from build123d import *

# Parameters (mm, degrees)
SKETCH5_W                = 5.15874
SKETCH5_H                = 60.071
SKETCH10_R               = 9.3345
BOSS_EXTRUDE1_DEPTH      = 31.75
CUT_EXTRUDE7_START       = 91.821
SKETCH8_R                = 12.7
CUT_EXTRUDE7_DEPTH       = 22.225
CUT_EXTRUDE9_DEPTH       = 93.765089454
CUT_EXTRUDE9_DEPTH_BACK  = 93.765089454
SKETCH11_W               = 2
SKETCH11_H               = 3
CUT_EXTRUDE10_DEPTH      = 93.765089454
CUT_EXTRUDE10_DEPTH_BACK = 93.765089454
SKETCH12_R               = 1.5875
CUT_EXTRUDE11_DEPTH      = 93.765089454
CUT_EXTRUDE11_DEPTH_BACK = 93.765089454
SKETCH13_R               = 1.5875


with BuildPart() as part:
    # Sketch5 → Revolve2 (revolve)
    with BuildSketch(Plane(origin=(0, 0, 0), x_dir=(1, 0, 0), z_dir=(0, 1, 0)), mode=Mode.PRIVATE) as revolve2_sk:
        with Locations((2.57937, -30.0355)):
            Rectangle(SKETCH5_W, SKETCH5_H)
    revolve(revolve2_sk.sketch.rotate(Axis((0, 0, 0), (0, 0, 1)), 180), axis=Axis((0, 0, 0), (0, 0, 1)))

    # Sketch10 → Boss-Extrude1 (add)
    with BuildSketch(Plane.XY.offset(60.071)):
        Circle(SKETCH10_R)
    extrude(amount=BOSS_EXTRUDE1_DEPTH)

    # Sketch8 → Cut-Extrude7 (cut)
    with BuildSketch(Plane.XY.offset(CUT_EXTRUDE7_START)):
        Circle(SKETCH8_R)
        Polygon((9.235721046, -0.808020891), (8.681700155, -0.254), (8.681700155, 0.254), (9.235721046, 0.808020891), (8.593912259, 1.257420242), (8.505698985, 1.75770258), (8.955098336, 2.399511367), (8.245002688, 2.730634406), (8.071256455, 3.207998257), (8.402379494, 3.918093905), (7.645572882, 4.120879625), (7.391572882, 4.56082053), (7.594358603, 5.317627141), (6.813836213, 5.385914002), (6.487300108, 5.775064579), (6.555586968, 6.555586968), (5.775064579, 6.487300108), (5.385914002, 6.813836213), (5.317627141, 7.594358603), (4.56082053, 7.391572882), (4.120879625, 7.645572882), (3.918093905, 8.402379494), (3.207998257, 8.071256455), (2.730634406, 8.245002688), (2.399511367, 8.955098336), (1.75770258, 8.505698985), (1.257420242, 8.593912259), (0.808020891, 9.235721046), (0.254, 8.681700155), (-0.254, 8.681700155), (-0.808020891, 9.235721046), (-1.257420242, 8.593912259), (-1.75770258, 8.505698985), (-2.399511367, 8.955098336), (-2.730634406, 8.245002688), (-3.207998257, 8.071256455), (-3.918093905, 8.402379494), (-4.120879625, 7.645572882), (-4.56082053, 7.391572882), (-5.317627141, 7.594358603), (-5.385914002, 6.813836213), (-5.775064579, 6.487300108), (-6.555586968, 6.555586968), (-6.487300108, 5.775064579), (-6.813836213, 5.385914002), (-7.594358603, 5.317627141), (-7.391572882, 4.56082053), (-7.645572882, 4.120879625), (-8.402379494, 3.918093905), (-8.071256455, 3.207998257), (-8.245002688, 2.730634406), (-8.955098336, 2.399511367), (-8.505698985, 1.75770258), (-8.593912259, 1.257420242), (-9.235721046, 0.808020891), (-8.681700155, 0.254), (-8.681700155, -0.254), (-9.235721046, -0.808020891), (-8.593912259, -1.257420242), (-8.505698985, -1.75770258), (-8.955098336, -2.399511367), (-8.245002688, -2.730634406), (-8.071256455, -3.207998257), (-8.402379494, -3.918093905), (-7.645572882, -4.120879625), (-7.391572882, -4.56082053), (-7.594358603, -5.317627141), (-6.813836213, -5.385914002), (-6.487300108, -5.775064579), (-6.555586968, -6.555586968), (-5.775064579, -6.487300108), (-5.385914002, -6.813836213), (-5.317627141, -7.594358603), (-4.56082053, -7.391572882), (-4.120879625, -7.645572882), (-3.918093905, -8.402379494), (-3.207998257, -8.071256455), (-2.730634406, -8.245002688), (-2.399511367, -8.955098336), (-1.75770258, -8.505698985), (-1.257420242, -8.593912259), (-0.808020891, -9.235721046), (-0.254, -8.681700155), (0.254, -8.681700155), (0.808020891, -9.235721046), (1.257420242, -8.593912259), (1.75770258, -8.505698985), (2.399511367, -8.955098336), (2.730634406, -8.245002688), (3.207998257, -8.071256455), (3.918093905, -8.402379494), (4.120879625, -7.645572882), (4.56082053, -7.391572882), (5.317627141, -7.594358603), (5.385914002, -6.813836213), (5.775064579, -6.487300108), (6.555586968, -6.555586968), (6.487300108, -5.775064579), (6.813836213, -5.385914002), (7.594358603, -5.317627141), (7.391572882, -4.56082053), (7.645572882, -4.120879625), (8.402379494, -3.918093905), (8.071256455, -3.207998257), (8.245002688, -2.730634406), (8.955098336, -2.399511367), (8.505698985, -1.75770258), (8.593912259, -1.257420242), align=None, mode=Mode.SUBTRACT)
    extrude(amount=-CUT_EXTRUDE7_DEPTH, mode=Mode.SUBTRACT)

    # Sketch11 → Cut-Extrude9 (cut, two sides: drawn at the far end of the back side and taken through both)
    with BuildSketch(Plane(origin=(0, 0, 0), x_dir=(1, 0, 0), z_dir=(0, 1, 0)).offset(-CUT_EXTRUDE9_DEPTH_BACK)):
        with Locations((0, -1.5)):
            Rectangle(SKETCH11_W, SKETCH11_H)
    extrude(amount=CUT_EXTRUDE9_DEPTH + CUT_EXTRUDE9_DEPTH_BACK, mode=Mode.SUBTRACT)

    # Sketch12 → Cut-Extrude10 (cut, two sides: drawn at the far end of the back side and taken through both)
    with BuildSketch(Plane(origin=(0, 0, 0), x_dir=(1, 0, 0), z_dir=(0, 1, 0)).offset(-CUT_EXTRUDE10_DEPTH_BACK)):
        with Locations(Location((0, -50.2285, 0), (0, 0, 270))):
            Circle(SKETCH12_R)
    extrude(amount=CUT_EXTRUDE10_DEPTH + CUT_EXTRUDE10_DEPTH_BACK, mode=Mode.SUBTRACT)

    # Sketch13 → Cut-Extrude11 (cut, two sides: drawn at the far end of the back side and taken through both)
    with BuildSketch(Plane(origin=(0, 0, 0), x_dir=(0, 0, -1), z_dir=(1, 0, 0)).offset(-CUT_EXTRUDE11_DEPTH_BACK)):
        with Locations((-56.261, 0)):
            Circle(SKETCH13_R)
    extrude(amount=CUT_EXTRUDE11_DEPTH + CUT_EXTRUDE11_DEPTH_BACK, mode=Mode.SUBTRACT)


solid = part.part
Work out the finished part from the listing and answer in its coordinate system (mm). A direction names the side the tool comes from. Coordinates: 2 decimals unless noted, no trailing zeros. Write each loop counter-clockwise with the first axis right and the second up, starting at its lowest first coordinate (ties: lowest second). Pieces come first, ordered by that corner, then holes.
1. Flat-ended cylindrical pins translate along their axes: pin 1 (2 mm diameter, centred on y = 4.5, z = 47, fed in from +X); pin 2 (10 mm diameter, centred on y = 3.5, z = 16.5, fed in from -X); pin 3 (6 mm diameter, centred on y = -3.5, z = 80, fed in from -X). Find the tip coordinate at first contact, or state that the pin passes through.
Results list:
pin 1: stops at x = 3.79
pin 2: stops at x = -5.16
pin 3: stops at x = -9.24
2. For faces 1 (the flat face through (4, -4, 60.071)), 2 (the flat face through (1, 0, 2)), 3 (the flat face through (3, 0, 0)), determine the directions among +Z, -Z, +X, -X, +Y, -Y from which every point of the face is accessible in a straight line to the end or side of a thin tool.
Results list:
face 1: -Z
face 2: -Z, +Y, -Y
face 3: -Z, +X, -X, +Y, -Y
3. For a pull along X with two mould halves and no side action, classify faces 4 (the cylindrical face through (0.07, -0.072, 48.643)), 5 (the cylindrical face through (-2.38, 4.577, 29.615)), 6 (the cylindrical face through (-0.072, 0.07, 57.847)) as +X half, -X half, draft (parallel to the pull), parting line (faces both ways), or undercut.
Results list:
face 4: undercut
face 5: parting line
face 6: draft
4. Consider line 1 along Z through (x, y) = (0, 0); line 2 along Z through (x, y) = (0, 1); line 3 along Z through (x, y) = (2.5, -6.5). Determine where each line is inside the solid, lowest interval first.
Results list:
line 1: z = 3 to 48.64, 51.82 to 54.67, 57.85 to 91.82
line 2: z = 3 to 48.64, 51.82 to 55.03, 57.49 to 91.82
line 3: z = 60.07 to 91.82
5. The part is cut by section A-A, the plane z = 17. Write down the section's boundary in (x, y).
Results list:
outline: circle Ø10.32 at (0, 0)
